Verification items for the finished model (mm, model axes). A direction names the side the tool comes from. Give positions to 0.01 mm unless a question says otherwise; leave off trailing zeros. Loops run counter-clockwise (first coordinate to the right, second up) from the corner with the lowest first, then second, coordinate; pieces in that order, holes last. Notation, with made-up numbers: (75.5, 20.5) - (128.5, 20.5) arc R27 ccw to (128.5, 36.5) - close; hole circle Ø3 at (11, -3). An arc over 180 degrees is marked (long way). One line per item, written item: value. Start each with the question number.
1. Sectioned sample at D-D (y = 0). Record the cut outline in (x, z).
2. Gauge pin test, flat ends, axial feed: pin 1 (3.5 mm diameter, centred on x = 0, z = 10.5, fed in from -Y); pin 2 (3 mm diameter, centred on y = -0.5, z = 10.5, fed in from -X); pin 3 (6 mm diameter, centred on y = 3.5, z = 4.5, fed in from +X); pin 4 (1.5 mm diameter, centred on y = 15.5, z = 12, fed in from -X). Record the tip position at first contact, or that the pin passes through.
3. Scan lines: L1, parallel to Y at x = 0, z = 0.65; L2, parallel to Z at x = 0, y = -10.85; L3, parallel to Z at x = -11, y = -9. Record each from-to range of solid material in increasing order. Write a range as [from, to].
4. Sectioned sample at B-B (z = 14.75). Record the cut outline in (x, y).
5. Sectioned sample at C-C (y = 9.5). Record the cut outline in (x, z), plus the area to 3 significant figures.
6. Access from +Z, -Z, +X, -X, +Y, -Y to the whole of each face (thin tool, end or side, straight path). Record for faces 4 (the flat face through (0, 0, 1)), 5 (the flat face through (0, -9, 16)), 6 (the cylindrical face through (-1.81, -8.15, 10.42)).
7. Sectioned sample at A-A (x = 0). Record the cut outline in (y, z), plus the area to 3 significant figures.
8. Mould release check, pull along Y, two halves, no side actions. Record for faces 1 (the cylindrical face through (1.68, 12.794, 0.493)), 2 (the cylindrical face through (0.07, -10.74, 8.9)), 3 (the cylindrical face through (-4.336, -19.524, 2.465)): pulls with the +Y half, pulls with the -Y half, needs draft (parallel to the pull), parting line crosses it, or undercut.
from build123d import *

# Parameters (mm, degrees)
CROQUIS1_R              = 20
SALIENTE_EXTRUIR1_DEPTH = 5
CROQUIS2_R              = 13.35
CROQUIS2_R_2            = 8.35
SALIENTE_EXTRUIR2_DEPTH = 11
CROQUIS3_R              = 1.6
CORTAR_EXTRUIR1_DEPTH   = 20
CROQUIS4_R              = 12.903487901
CORTAR_EXTRUIR3_DEPTH   = 1


with BuildPart() as part:
    # Croquis1 → Saliente-Extruir1 (new body)
    with BuildSketch(Plane.XY):
        Circle(CROQUIS1_R)
    extrude(amount=SALIENTE_EXTRUIR1_DEPTH)

    # Croquis2 → Saliente-Extruir2 (add)
    with BuildSketch(Plane.XY.offset(5)):
        Circle(CROQUIS2_R)
        Circle(CROQUIS2_R_2, mode=Mode.SUBTRACT)
    extrude(amount=SALIENTE_EXTRUIR2_DEPTH)

    # Croquis3 → Cortar-Extruir1 (cut, symmetric)
    with BuildSketch(Plane(origin=(0, 0, 0), x_dir=(1, 0, 0), z_dir=(0, 1, 0))):
        with Locations(Location((0, -10.5, 0), (0, 0, 270))):
            Circle(CROQUIS3_R)
    extrude(amount=CORTAR_EXTRUIR1_DEPTH, both=True, mode=Mode.SUBTRACT)

    # Croquis4 → Cortar-Extruir3 (cut)
    with BuildSketch(Plane(origin=(0, 0, 0), x_dir=(-1, 0, 0), z_dir=(0, 0, -1))):
        Circle(CROQUIS4_R)
    extrude(amount=-CORTAR_EXTRUIR3_DEPTH, mode=Mode.SUBTRACT)


solid = part.part
Results are:
1. outline: (-20, 0) - (-12.9, 0) - (-12.9, 1) - (12.9, 1) - (12.9, 0) - (20, 0) - (20, 5) - (13.35, 5) - (13.35, 16) - (8.35, 16) - (8.35, 5) - (-8.35, 5) - (-8.35, 16) - (-13.35, 16) - (-13.35, 5) - (-20, 5) - close
2. pin 1: stops at y = -13.35
2. pin 2: stops at x = -13.35
2. pin 3: stops at x = 19.99
2. pin 4: passes through
3. L1: y = [-20, -12.9], [12.9, 20]
3. L2: z = [1, 8.9], [12.1, 16]
3. L3: z = [0, 5]
4. outline: circle Ø26.7 at (0, 0); hole circle Ø16.7 at (0, 0)
5. outline: (-17.6, 0) - (-8.73, 0) - (-8.73, 1) - (8.73, 1) - (8.73, 0) - (17.6, 0) - (17.6, 5) - (9.38, 5) - (9.38, 16) - (-9.38, 16) - (-9.38, 5) - (-17.6, 5) - close; hole circle Ø3.2 at (0, 10.5)
5. area: 357 mm^2
6. face 4: -Z
6. face 5: +Z, +X, -X, +Y, -Y
6. face 6: +Z
7. outline: (-20, 0) - (-12.9, 0) - (-12.9, 1) - (12.9, 1) - (12.9, 0) - (20, 0) - (20, 5) - (13.35, 5) - (13.35, 8.9) - (8.35, 8.9) - (8.35, 5) - (-8.35, 5) - (-8.35, 8.9) - (-13.35, 8.9) - (-13.35, 5) - (-20, 5) - close; (-13.35, 12.1) - (-8.35, 12.1) - (-8.35, 16) - (-13.35, 16) - close; (8.35, 12.1) - (13.35, 12.1) - (13.35, 16) - (8.35, 16) - close
7. area: 252 mm^2
8. face 1: undercut
8. face 2: needs draft
8. face 3: parting line crosses it
